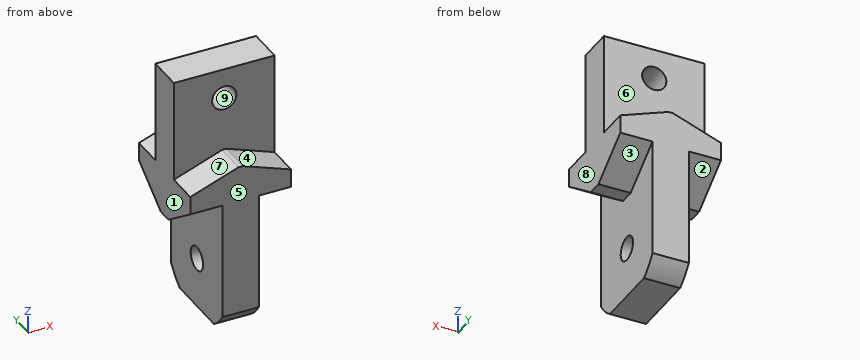
from build123d import *

# Parameters (mm, degrees)
SKETCH_1_W               = 25
SKETCH_1_H               = 25
EXTRUDE_1_DEPTH          = 68.359061336
SKETCH_2_W               = 25
SKETCH_2_H               = 8
CUT_EXTRUDE_3_DEPTH      = 26
CUT_EXTRUDE_START        = -17
SKETCH_4_R               = 3
CUT_EXTRUDE_4_DEPTH      = 57
MOVE_BODY_1_ANGLE        = 90
SKETCH_5_W               = 25
SKETCH_5_H               = 25
EXTRUDE_2_DEPTH          = 10
SKETCH_9_W               = 25
SKETCH_9_H               = 9
CUT_EXTRUDE_8_DEPTH      = 5
CUT_EXTRUDE_5_DEPTH      = 8
MIRROR_8_COPY_1_DEPTH    = 8
CUT_EXTRUDE_START_2      = 10
SKETCH_8_R               = 3
CUT_EXTRUDE_6_DEPTH      = 10
MIRROR_START             = 10
MIRROR_7_COPY_1_SKETCH_R = 3
MIRROR_7_COPY_1_DEPTH    = 10
CUT_EXTRUDE_9_DEPTH      = 10


# Read off the part's stored shape, not the designer's step: the other step
with BuildPart() as part:
    # Sketch 1 → Extrude 1 (new body)
    with BuildSketch(Plane.XY):
        Rectangle(SKETCH_1_W, SKETCH_1_H)
    extrude(amount=-EXTRUDE_1_DEPTH)

    # Sketch 2 → Cut-Extrude 3 (cut)
    with BuildSketch(Plane(origin=(0, 0, -68.359061336), x_dir=(-1, 0, 0), z_dir=(0, 0, -1))):
        with Locations((0, 8.5)):
            Rectangle(SKETCH_2_W, SKETCH_2_H)
        with Locations((0, -8.5)):
            Rectangle(SKETCH_2_W, SKETCH_2_H)
    cut_extrude_3 = extrude(amount=-CUT_EXTRUDE_3_DEPTH, mode=Mode.SUBTRACT)

    # Sketch 4 → Cut-Extrude 4 (cut)
    with BuildSketch(Plane.XZ.offset(-4.5).offset(CUT_EXTRUDE_START)):
        with Locations(Location((0, -55.859061336, 0), (0, 0, 90))):
            Circle(SKETCH_4_R)
    cut_extrude_4 = extrude(amount=CUT_EXTRUDE_4_DEPTH, mode=Mode.SUBTRACT)

    # Mirror 4: Cut-Extrude 3, Cut-Extrude 4 across plane
    add(cut_extrude_3.mirror(Plane.XY.offset(-34.179530668)), mode=Mode.SUBTRACT)
    add(cut_extrude_4.mirror(Plane.XY.offset(-34.179530668)), mode=Mode.SUBTRACT)


with BuildPart() as body_2:
    # Other 1: the piece on the far side of the plane
    add(part.part)
    split(bisect_by=Plane.XY.offset(-34.179530668), keep=Keep.BOTTOM)


with BuildPart() as part_1:
    add(part.part)

    # Other 1
    split(bisect_by=Plane.XY.offset(-34.179530668), keep=Keep.TOP)



with BuildPart() as body_2_1:
    # Move Body 1: moved
    add(body_2.part.rotate(Axis((0, 0, 0), (0, 0, 1)), MOVE_BODY_1_ANGLE))


with BuildPart() as part_2:
    add(part_1.part)

    add(body_2_1.part)  # Extrude 2 merges body 2
    # Sketch 5 → Extrude 2 (add)
    with BuildSketch(Plane(origin=(0, 0, -42.359061336), x_dir=(-1, 0, 0), z_dir=(0, 0, -1))):
        Rectangle(SKETCH_5_W, SKETCH_5_H)
    extrude(amount=-EXTRUDE_2_DEPTH)

    # Sketch 9 → Cut-Extrude 8 (cut)
    with BuildSketch(Plane.XY):
        Rectangle(SKETCH_9_W, SKETCH_9_H)
    extrude(amount=-CUT_EXTRUDE_8_DEPTH, mode=Mode.SUBTRACT)

    # Sketch 7 → Cut-Extrude 5 (cut)
    with BuildSketch(Plane(origin=(-8, 4.5, 0), x_dir=(0, 0, 1), z_dir=(0, -1, 0))):
        Polygon((7.793639977, -63.756317597), (-41.547874973, 71.808380572), (-55.762350506, 74.314776125), (-6.420835555, -61.249922044), align=None)
    cut_extrude_5 = extrude(amount=-CUT_EXTRUDE_5_DEPTH, mode=Mode.SUBTRACT)

    # Mirror 5: Cut-Extrude 5 across plane
    add(cut_extrude_5.mirror(Plane(origin=(0, 0, 0), x_dir=(0, 0, 1), z_dir=(1, 0, 0))), mode=Mode.SUBTRACT)

    # Mirror 8: Cut-Extrude 5 across plane
    add(cut_extrude_5.mirror(Plane(origin=(0, 0, 0), x_dir=(0, 0, 1), z_dir=(0, -1, 0))), mode=Mode.SUBTRACT)

    # Mirror 8 copy 1 sketch → Mirror 8 copy 1 (cut)
    with BuildSketch(Plane(origin=(8, -4.5, 0), x_dir=(0, 0, 1), z_dir=(0, 1, 0))):
        Polygon((7.793639977, -63.756317597), (-41.547874973, 71.808380572), (-55.762350506, 74.314776125), (-6.420835555, -61.249922044), align=None)
    extrude(amount=-MIRROR_8_COPY_1_DEPTH, mode=Mode.SUBTRACT)

    # Sketch 8 → Cut-Extrude 6 (cut)
    with BuildSketch(Plane(origin=(-4.5, 0, 0), x_dir=(0, 1, 0), z_dir=(-1, 0, 0)).offset(CUT_EXTRUDE_START_2)):
        Polygon((26.984001119, 62.545716444), (-15.512472392, 32.789365343), (-26.984001119, 49.172406229), (15.512472392, 78.92875733), align=None)
        with Locations(Location((0, 55.859061336, 0), (0, 0, 270))):
            Circle(SKETCH_8_R, mode=Mode.SUBTRACT)
    cut_extrude_6 = extrude(amount=-CUT_EXTRUDE_6_DEPTH, mode=Mode.SUBTRACT)

    # Mirror 6: Cut-Extrude 6 across plane
    add(cut_extrude_6.mirror(Plane(origin=(0, 0, 0), x_dir=(0, 0, 1), z_dir=(1, 0, 0))), mode=Mode.SUBTRACT)

    # Mirror 7: Cut-Extrude 6 across plane
    add(cut_extrude_6.mirror(Plane.ZX), mode=Mode.SUBTRACT)

    # Mirror 7 copy 1 sketch → Mirror 7 copy 1 (cut)
    with BuildSketch(Plane(origin=(4.5, 0, 0), x_dir=(0, -1, 0), z_dir=(1, 0, 0)).offset(MIRROR_START)):
        Polygon((26.984001119, 62.545716444), (-15.512472392, 32.789365343), (-26.984001119, 49.172406229), (15.512472392, 78.92875733), align=None)
        with Locations(Location((0, 55.859061336, 0), (0, 0, 270))):
            Circle(MIRROR_7_COPY_1_SKETCH_R, mode=Mode.SUBTRACT)
    extrude(amount=-MIRROR_7_COPY_1_DEPTH, mode=Mode.SUBTRACT)

    # Sketch 10 → Cut-Extrude 9 (cut)
    with BuildSketch(Plane.ZY.offset(4.5)):
        with BuildLine():
            Line((-64.150623312, 12.5), (-68.359061336, 12.5))
            Line((-68.359061336, 12.5), (-68.359061336, 8.291561976))
            ThreePointArc((-68.359061336, 8.291561976), (-66.465663054, 10.606601718), (-64.150623312, 12.5))
        make_face()
        with BuildLine():
            Line((-64.150623312, -12.5), (-68.359061336, -12.5))
            Line((-68.359061336, -12.5), (-68.359061336, -8.291561976))
            ThreePointArc((-68.359061336, -8.291561976), (-66.465663054, -10.606601718), (-64.150623312, -12.5))
        make_face()
    extrude(amount=-CUT_EXTRUDE_9_DEPTH, mode=Mode.SUBTRACT)


solid = part_2.part
For this review, take the finished solid that the model builds, in its own axes (mm). Face numbers are marked on the shaded views. A direction names the side the tool comes from. Round coordinates to 2 decimals unless told otherwise and drop trailing zeros. Write each loop counter-clockwise with the first axis right and the second up, starting at its lowest first coordinate (ties: lowest second). Pieces come first, ordered by that corner, then holes. Notation, with made-up numbers: (51.5, 32) -> (66.5, 32) arc R29 ccw to (66.5, 61) -> close; hole circle Ø9 at (89.5, 41.5). An arc over 180 degrees is marked (long way). Put each result on its own line as item: value.
Q1. The part is to be moulded in two halves that separate along X. For the marked faces 6, 7, 8 and 9, say which applies: released by +X, released by -X, zero draft, split by the parting line, or undercut.
Determined:
face 6: zero draft
face 7: released by -X
face 8: released by +X
face 9: undercut
Q2. Consider section C-C on x = 10.75. State the section outline as (y, z) points.
Determined:
outline: (-12.5, -34.9) -> (-1.85, -42.36) -> (1.85, -42.36) -> (12.5, -34.9) -> (12.5, -29.71) -> (4.5, -29.71) -> (4.5, -5) -> (-4.5, -5) -> (-4.5, -29.71) -> (-12.5, -29.71) -> close
Q3. Consider section A-A on y = 0. State the section outline as (x, z) points, and give its area (3 significant figures).
Determined:
outline: (-12.5, -42.36) -> (-4.5, -42.36) -> (-4.5, -52.86) -> (4.5, -52.86) -> (4.5, -42.36) -> (12.5, -42.36) -> (12.5, -5) -> (-12.5, -5) -> close; (-4.5, -68.36) -> (4.5, -68.36) -> (4.5, -58.86) -> (-4.5, -58.86) -> close; hole circle Ø6 at (0, -12.5)
area: 1,090 mm^2
Q4. Consider section B-B on z = -12.5. State the section outline as (x, y) points.
Determined:
outline: (-12.5, -4.5) -> (-3, -4.5) -> (-3, 4.5) -> (-12.5, 4.5) -> close; (3, -4.5) -> (12.5, -4.5) -> (12.5, 4.5) -> (3, 4.5) -> close
Q5. Consider section D-D on y = 7.5. State the section outline as (x, z) points.
Determined:
outline: (-12.5, -38.4) -> (-4.5, -38.4) -> (-4.5, -68.36) -> (4.5, -68.36) -> (4.5, -38.4) -> (12.5, -38.4) -> (12.5, -30.35) -> (0.54, -26) -> (-0.54, -26) -> (-12.5, -30.35) -> close
Q6. Clearance check with flat-ended pins moving along their axes: pin 1 Ø7.5 at (y, z) = (1, -59) entering from +X; pin 2 Ø1.2 at (x, y) = (0, 10) entering from +Z; pin 3 Ø4 at (x, y) = (-9.5, -1) entering from -Z. State where each tip first meets the part, or that it passes through.
Determined:
pin 1: stops at x = 4.5
pin 2: stops at z = -26
pin 3: stops at z = -42.36
Q7. Machinability: for the marked faces 1, 2, 3, 4 and 5, which of the approach directions +Z, -Z, +X, -X, +Y, -Y give a long, thin tool a straight path to every point of the face, cutting with its end or side? Answer none if there is none.
Determined:
face 1: +Z, -Z, -X, +Y, -Y
face 2: -Z, -X, +Y
face 3: -Z, +X, +Y
face 4: +Z, +X, -Y
face 5: +Z, -Z, +X, -X, -Y
Q8. To check wall thickness, follow L1, parallel to X at y = -1.5, z = -12.5; L2, parallel to X at y = -1.75, z = -45.5. State the ranges of each line that lie inside material, in increasing order. Write a range as [from, to].
Determined:
L1: x = [-12.5, -3], [3, 12.5]
L2: x = [-4.5, 4.5]
